```python
from build123d import *

# Parameters (mm, degrees)
F0_R     = 13.5
F1_DEPTH = 2.5
F2_R     = 6.075
F2_R_2   = 4.075
F3_DEPTH = 5
F4_R     = 2
F5_R     = 2


with BuildPart() as f1:
    # F0 (on Top) → F1 (new body)
    with BuildSketch(Plane.XY):
        Circle(F0_R)
    extrude(amount=F1_DEPTH)

    # F2 (on face) → F3 (join)
    with BuildSketch(Plane.XY.offset(2.5)):
        Circle(F2_R)
        Circle(F2_R_2, mode=Mode.SUBTRACT)
    extrude(amount=F3_DEPTH)

    # F4
    f4_edges = [f1.edges().sort_by_distance(p)[0] for p in [
        (-4.075, 0, 2.5),
    ]]
    fillet(f4_edges, radius=F4_R)

    # F5
    f5_edges = [f1.edges().sort_by_distance(p)[0] for p in [
        (-13.5, 0, 0),
    ]]
    fillet(f5_edges, radius=F5_R)


solid = f1.part
```
Geometry check sheet. Reference: the model listing, model coordinates, mm. A direction names the side the tool comes from. Round coordinates to 2 decimals unless told otherwise and drop trailing zeros. Order: outer loops, then holes, each group sorted by start corner. A loop starts at its lowest first (then second) coordinate and runs counter-clockwise, first axis right, second up. Notation, with made-up numbers: (12, -32.5) - (64, -32.5) arc R23 ccw to (64, -23.5) - close; hole circle Ø4 at (25.25, 18.5). An arc over 180 degrees is marked (long way). Use a Markdown table: item, result. Add a question column.
1) Section check A-A (y = 0). Record the cut outline in (x, z) (3 decimals), then the cut area to 3 significant figures.
2) Thickness scan on line 1 along Y through (x, z) = (0, 6.2) (3 decimals); line 2 along X through (y, z) = (0.5, 4); line 3 along Z through (x, y) = (-7, -6.25). Record the ranges inside material, lowest first.
3) Section check C-C (z = 1.5). Record the cut outline in (x, y).
4) Mould release check, pull along Y, two halves, no side actions. Record for faces 1 (the cylindrical face through (-1.32, -5.93, 4.96)), 2 (the flat face through (0, 0, 0)), 3 (the cylindrical face through (-3.234, -2.48, 5.979)): released by +Y, released by -Y, zero draft, split by the parting line, or undercut.
5) Gauge pin test, flat ends, axial feed: P1, Ø4.5, axis at x = 0.5, y = 1, coming from the +Z side; P2, Ø1.5, axis at x = 8, z = 2.5, coming from the -Y side; P3, Ø1.5, axis at x = -10, y = 6.5, coming from the +Z side. Record the tip position at first contact, or that the pin passes through.
6) Set-up check for faces 4 (the flat face through (6, -3, 2.5)), 5 (the flat face through (-1.4, -4, 7.5)): record each of +Z, -Z, +X, -X, +Y, -Y from which the full face is reachable in a straight line by a thin tool's end or side.
Established:
| question | item | result |
|---|---|---|
| 1 | outline | (-13.5, 2) arc R2 ccw to (-11.5, 0) - (11.5, 0) arc R2 ccw to (13.5, 2) - (13.5, 2.5) - (6.075, 2.5) - (6.075, 7.5) - (4.075, 7.5) - (4.075, 4.5) arc R2 cw to (2.075, 2.5) - (-2.075, 2.5) arc R2 cw to (-4.075, 4.5) - (-4.075, 7.5) - (-6.075, 7.5) - (-6.075, 2.5) - (-13.5, 2.5) - close |
| 1 | area | 87.5 mm2 |
| 2 | line 1 | -6.075 to -4.075, 4.075 to 6.075 |
| 2 | line 2 | -6.05 to -3.98, 3.98 to 6.05 |
| 2 | line 3 | 0 to 2.5 |
| 3 | outline | circle Ø26.87 at (0, 0) |
| 4 | face 1 | split by the parting line |
| 4 | face 2 | zero draft |
| 4 | face 3 | undercut |
| 5 | P1 | z = 2.97 |
| 5 | P2 | y = -11.39 |
| 5 | P3 | z = 2.5 |
| 6 | face 4 | +Z |
| 6 | face 5 | +Z, +X, -X, +Y, -Y |
